Work out the finished part from the listing and answer in its coordinate system (mm). Round coordinates to 2 decimals unless told otherwise and drop trailing zeros. Order: outer loops, then holes, each group sorted by start corner. A loop starts at its lowest first (then second) coordinate and runs counter-clockwise, first axis right, second up. Notation, with made-up numbers: (-9, 38.5) - (5, 38.5) arc R18 cw to (5, 61.5) - close; hole circle Ø11 at (-39.75, 16). An arc over 180 degrees is marked (long way). Put each result on its own line as item: value.
Autodesk Inventor part; units mm, degrees
ref_plane "YZ Plane" through (0, 0, 0) normal (1, 0, 0) x (0, 1, 0)
ref_plane "XZ Plane" through (0, 0, 0) normal (0, 1, 0) x (-1, 0, 0)
ref_plane "XY Plane" through (0, 0, 0) normal (0, 0, 1) x (1, 0, 0)
sketch "Sketch1" plane through (0, 0, 0) normal (0, 0, 1) x (1, 0, 0)
  line L0 (-64.9406, 96.6023) -> (189.0594, 96.6023)
  line L1 (189.0594, 96.6023) -> (189.0594, -792.3977)
  line L2 (189.0594, -792.3977) -> (-64.9406, -792.3977)
  line L3 (-64.9406, -792.3977) -> (-64.9406, 96.6023)
  line L4 (-64.9406, 96.6023) -> (87.4594, 96.6023)
  line L5 (87.4594, 96.6023) -> (87.4594, -364.1537)
  line L6 (87.4594, -364.1537) -> (-64.9406, -364.1537)
  line L7 (-64.9406, -364.1537) -> (-64.9406, 96.6023)
  point P0 (0, 0)
  dimension "d0" = 254
  dimension "d1" = 889
  dimension "d2" = 152.4
  dimension "d3" = 460.756
extrude "Extrusion1" add sketch "Sketch1" along normal blind 6.35 contours L0 L1 L2 L3 L6 L5
sketch "Sketch2" plane through (-64.9406, -792.3977, 0) normal (-1, 0, 0) x (0, 0, 1)
  line L0 (6.35, 428.244) -> (0, 428.244)
  line L1 (0, 428.244) -> (0, 0)
  line L2 (0, 0) -> (6.35, 0)
  line L3 (6.35, 0) -> (6.35, 428.244)
  point P0 (0, 792.3977)
extrude "Extrusion2" add sketch "Sketch2" along normal blind 6.35
sketch "Sketch3" plane through (0, 0, 6.35) normal (0, 0, 1) x (1, 0, 0)
  line L0 (87.4594, 96.6023) -> (189.0594, 96.6023)
  line L1 (87.4594, -364.1537) -> (90.6344, -364.1537)
  line L2 (90.6344, -364.1537) -> (90.6344, 96.6023)
  line L3 (90.6344, 96.6023) -> (87.4594, 96.6023)
  line L4 (87.4594, 96.6023) -> (87.4594, -364.1537)
  point P0 (0, 0)
  dimension "d8" = 3.175
extrude "Extrusion3" cut sketch "Sketch3" against normal blind 6.35
sketch "Sketch4" plane through (189.0594, 96.6023, 6.35) normal (0, 1, 0) x (1, 0, 0)
  line L0 (-98.425, 6.35) -> (-98.425, 0)
  line L1 (-98.425, 0) -> (0, 0)
  line L2 (0, 6.35) -> (0, 0)
  line L3 (0, 6.35) -> (-98.425, 6.35)
  point P0 (-189.0594, 6.35)
extrude "Extrusion4" add sketch "Sketch4" along normal blind 6.35
sketch "Sketch5" plane through (189.0594, 102.9523, 6.35) normal (0, 1, 0) x (1, 0, 0)
  line L0 (-98.425, 6.35) -> (0, 6.35)
  line L1 (-98.425, 0) -> (-98.425, 6.35)
  line L2 (0, 0) -> (-98.425, 0)
  line L3 (0, 6.35) -> (0, 0)
  point P0 (-189.0594, 6.35)
extrude "Extrusion5" cut sketch "Sketch5" against normal blind 6.35
sketch "Sketch6" plane through (189.0594, 96.6023, 6.35) normal (0, 1, 0) x (1, 0, 0)
  line L0 (-98.425, 0) -> (-98.425, 6.35)
  line L1 (0, 0) -> (-98.425, 0)
  line L2 (0, 6.35) -> (0, 0)
  line L3 (-98.425, 6.35) -> (0, 6.35)
  point P0 (-189.0594, 6.35)
extrude "Extrusion6" add sketch "Sketch6" along normal blind 6.35
sketch "Sketch7" plane through (0, 0, 6.35) normal (0, 0, 1) x (1, 0, 0)
  line L0 (90.6344, -364.1537) -> (-71.2906, -364.1537)
  line L1 (-71.2906, -364.1537) -> (-71.2906, -792.3977)
  line L2 (189.0594, -792.3977) -> (-71.2906, -792.3977)
  line L3 (189.0594, 102.9523) -> (189.0594, -792.3977)
  line L4 (189.0594, 102.9523) -> (90.6344, 102.9523)
  line L5 (0, -364.1537) -> (0, -688.0037)
  line L6 (0, -688.0037) -> (-71.2906, -688.0037)
  line L7 (0, -688.0037) -> (189.0594, -688.0037)
  point P0 (0, 0)
  dimension "d17" = 323.85
extrude "Extrusion7" cut sketch "Sketch7" against normal blind 25.4 contours L7 L3 L2 L1 L6
sketch "Sketch8" plane through (0, 0, 0) normal (0, 0, -1) x (-1, 0, 0)
  line L0 (71.2906, -688.0037) -> (71.2906, -364.1537)
  line L1 (-90.6344, -364.1537) -> (71.2906, -364.1537)
  line L2 (71.2906, -364.1537) -> (71.2906, -376.8537)
  line L3 (71.2906, -376.8537) -> (-90.6344, -376.8537)
  line L4 (-90.6344, -376.8537) -> (-90.6344, -364.1537)
  point P0 (0, 0)
  dimension "d20" = 12.7
extrude "Extrusion8" cut sketch "Sketch8" against normal blind 25.4
sketch "Sketch9" plane through (0, 0, 6.35) normal (0, 0, 1) x (1, 0, 0)
  line L0 (-71.2906, -376.8537) -> (-64.9406, -376.8537)
  line L1 (-64.9406, -376.8537) -> (-64.9406, -364.1537)
  line L2 (-64.9406, -364.1537) -> (-71.2906, -364.1537)
  line L3 (-71.2906, -364.1537) -> (-71.2906, -376.8537)
  point P0 (0, 0)
  dimension "d23" = 6.35
  dimension "d24" = 12.7
extrude "Extrusion9" add sketch "Sketch9" against normal blind 6.35
sketch "Sketch10" plane through (0, 0, 6.35) normal (0, 0, 1) x (1, 0, 0)
  line L0 (189.0594, 102.9523) -> (189.0594, -688.0037)
  line L1 (189.0594, 102.9523) -> (90.6344, 102.9523)
  line L2 (90.6344, 102.9523) -> (189.0594, 102.9523)
  line L3 (189.0594, 102.9523) -> (189.0594, 83.9023)
  line L4 (189.0594, 83.9023) -> (90.6344, 83.9023)
  line L5 (90.6344, 83.9023) -> (90.6344, 102.9523)
  point P0 (0, 0)
  dimension "d27" = 19.05
extrude "Extrusion10" cut sketch "Sketch10" against normal blind 6.35
properties part number "side"
1) Straight lines are drawn through the part: L1, parallel to Y at x = 52, z = 3; L2, parallel to X at y = -303.5, z = 0.5. For each, find the intervals that lie inside material, in ascending order. Write a range as from..to.
Findings below:
L1: y = -688..-376.85
L2: x = 90.63..189.06
2) Given pin 1 Ø3 at (x, z) = (28, 3) entering from +Y; pin 2 Ø3 at (y, z) = (-132, 2.5) entering from -X, each flat-ended and moving along its own axis, determine where each tip first touches the part or whether it passes through.
Findings below:
pin 1: stops at y = -376.85
pin 2: stops at x = 90.63
3) A cutting plane is placed at A-A on z = 2. Write down the section's boundary in (x, y), then the cut area to 3 significant figures.
Findings below:
outline: (-71.29, -688) - (189.06, -688) - (189.06, 83.9) - (90.63, 83.9) - (90.63, -376.85) - (-64.94, -376.85) - (-64.94, -364.15) - (-71.29, -364.15) - close
area: 126,000 mm2
4) A cutting plane is placed at C-C on x = -24. Write down the section's boundary in (y, z), then the cut area to 3 significant figures.
Findings below:
outline: (-688, 0) - (-376.85, 0) - (-376.85, 6.35) - (-688, 6.35) - close
area: 1,980 mm2
5) A cutting plane is placed at B-B on y = -116.5. Write down the section's boundary in (x, z), then the cut area to 3 significant figures.
Findings below:
outline: (90.63, 0) - (189.06, 0) - (189.06, 6.35) - (90.63, 6.35) - close
area: 625 mm2
